Could you check a few things on this model? Use its own coordinates, in mm. A direction names the side the tool comes from. Round coordinates to 2 decimals unless told otherwise and drop trailing zeros. Write each loop counter-clockwise with the first axis right and the second up, starting at its lowest first coordinate (ties: lowest second). Pieces come first, ordered by that corner, then holes. Notation, with made-up numbers: (30, 89) -> (71, 89) arc R33 cw to (71, 125) -> close; hole circle Ø2 at (-35, 52.5). An arc over 180 degrees is marked (long way). Answer in a Markdown table with one row per item.
from build123d import *

# Parameters (mm, degrees)
SKICA1_W                          = 144
SKICA1_H                          = 144
P_IDAT_VYSUNUT_M1_DEPTH           = 7
D_RY_PRO_KOL_K_VELIKOST_MM1_D     = 5.1
D_RY_PRO_KOL_K_VELIKOST_MM1_DEPTH = 6
ODEBRAT_VYSUNUT_M1_DEPTH          = 4
ODEBRAT_VYSUNUT_M2_DEPTH          = 102.901913623
ZAOBLIT1_R                        = 10


with BuildPart() as part:
    # Skica1 → Přidat vysunutím1 (new body)
    with BuildSketch(Plane.XY):
        Rectangle(SKICA1_W, SKICA1_H)
    extrude(amount=P_IDAT_VYSUNUT_M1_DEPTH)

    # Díry pro kolík, velikost mm1
    with Locations(Plane.XY.offset(7)):
        with Locations((-62.25, -62.25), (-62.25, 62.25), (62.25, 62.25), (62.25, -62.25)):
            Hole(D_RY_PRO_KOL_K_VELIKOST_MM1_D / 2, depth=D_RY_PRO_KOL_K_VELIKOST_MM1_DEPTH)

    # Skica5 → Odebrat vysunutím1 (cut)
    with BuildSketch(Plane.XY.offset(7)):
        Polygon((-70, -47), (-47, -70), (47, -70), (70, -47), (70, 47), (54.75233406, 62.24766594), (54.75233406, 72), (-54.75233406, 72), (-54.75233406, 62.24766594), (-70, 47), align=None)
    extrude(amount=-ODEBRAT_VYSUNUT_M1_DEPTH, mode=Mode.SUBTRACT)

    # Skica6 → Odebrat vysunutím2 (cut, through all)
    with BuildSketch(Plane.XY.offset(3)):
        with BuildLine():
            ThreePointArc((69.570557709, 5), (0, 69.75), (-69.570557709, 5))
            Line((-69.570557709, 5), (69.570557709, 5))
        make_face()
        with BuildLine():
            Line((69.570557709, -5), (-69.570557709, -5))
            ThreePointArc((-69.570557709, -5), (0, -69.75), (69.570557709, -5))
        make_face()
    extrude(amount=-ODEBRAT_VYSUNUT_M2_DEPTH, mode=Mode.SUBTRACT)

    # Zaoblit1
    zaoblit1_edges = [part.edges().sort_by_distance(p)[0] for p in [
        (72, -72, 3.5),
        (-72, -72, 3.5),
        (-72, 72, 3.5),
        (72, 72, 3.5),
    ]]
    fillet(zaoblit1_edges, radius=ZAOBLIT1_R)


solid = part.part
1) Imagine slicing it at B-B, the plane y = 22. Please give me the cut outline in (x, z), plus the area to 3 significant figures.
Findings:
| item | result |
|---|---|
| outline | (-72, 0) -> (-66.19, 0) -> (-66.19, 3) -> (-70, 3) -> (-70, 7) -> (-72, 7) -> close; (66.19, 0) -> (72, 0) -> (72, 7) -> (70, 7) -> (70, 3) -> (66.19, 3) -> close |
| area | 50.9 mm^2 |
2) Thinking about a two-plate mould opening in X: for faces 4 (the face through (10, 0, 0)), 5 (the face through (-72, -1, 3)), 6 (the face through (-59.702, -62.138, 3.958)), which applies, +X half, -X half, draft (parallel to the pull), parting line (faces both ways), or undercut?
Findings:
| item | result |
|---|---|
| face 4 | draft |
| face 5 | -X half |
| face 6 | undercut |
3) Imagine slicing it at D-D, the plane x = -20. Please give me the cut outline in (y, z), plus the area to 3 significant figures.
Findings:
| item | result |
|---|---|
| outline | (-72, 0) -> (-66.82, 0) -> (-66.82, 3) -> (-70, 3) -> (-70, 7) -> (-72, 7) -> close; (-5, 0) -> (5, 0) -> (5, 3) -> (-5, 3) -> close; (66.82, 0) -> (72, 0) -> (72, 3) -> (66.82, 3) -> close |
| area | 69.1 mm^2 |
4) Please list where these lines run through material, in increasing order: line 1 (Y direction, x = 62.25, z = 5.45); line 2 (Y direction, x = -43, z = 0.5).
Findings:
| item | result |
|---|---|
| line 1 | y = -72 to -64.8, -59.7 to -54.75, 54.75 to 59.7, 64.8 to 72 |
| line 2 | y = -72 to -54.92, -5 to 5, 54.92 to 72 |
5) For pin 1 (2 mm diameter, centred on x = 11, z = 5.5, fed in from +Y); pin 2 (2.5 mm diameter, centred on x = -62, y = 63, fed in from +Z), each with a flat end and sliding along its axis, tell me the tip position at first contact or that it passes through.
Findings:
| item | result |
|---|---|
| pin 1 | stops at y = -70 |
| pin 2 | stops at z = 1 |
6) Imagine slicing it at C-C, the plane x = -1.5. Please give me the cut outline in (y, z), plus the area to 3 significant figures.
Findings:
| item | result |
|---|---|
| outline | (-72, 0) -> (-69.73, 0) -> (-69.73, 3) -> (-70, 3) -> (-70, 7) -> (-72, 7) -> close; (-5, 0) -> (5, 0) -> (5, 3) -> (-5, 3) -> close; (69.73, 0) -> (72, 0) -> (72, 3) -> (69.73, 3) -> close |
| area | 51.6 mm^2 |
7) For faces 1 (the face through (62, 62, 1)), 2 (the face through (-54.752, 67, 5)), 3 (the face through (68.99, -69.15, 3.55)), which set-ups out of +Z, -Z, +X, -X, +Y, -Y let a thin tool reach every point of the face, with its end or its side?
Findings:
| item | result |
|---|---|
| face 1 | +Z |
| face 2 | +Z, +Y |
| face 3 | +Z, -Z, +X, -Y |
8) Imagine slicing it at A-A, the plane z = 5.75. Please give me the cut outline in (x, y), plus the area to 3 significant figures.
Findings:
| item | result |
|---|---|
| outline | (-72, -62) arc R10 ccw to (-62, -72) -> (62, -72) arc R10 ccw to (72, -62) -> (72, 62) arc R10 ccw to (62, 72) -> (54.75, 72) -> (54.75, 62.25) -> (70, 47) -> (70, -47) -> (47, -70) -> (-47, -70) -> (-70, -47) -> (-70, 47) -> (-54.75, 62.25) -> (-54.75, 72) -> (-62, 72) arc R10 ccw to (-72, 62) -> close; hole circle Ø5.1 at (-62.25, -62.25); hole circle Ø5.1 at (-62.25, 62.25); hole circle Ø5.1 at (62.25, -62.25); hole circle Ø5.1 at (62.25, 62.25) |
| area | 1,750 mm^2 |
